Can you work these out from the model? Positions are in its coordinate system, mm. A direction names the side the tool comes from. Round coordinates to 2 decimals unless told otherwise and drop trailing zeros. Loops run counter-clockwise (first coordinate to the right, second up) from the corner with the lowest first, then second, coordinate; pieces in that order, holes last. Notation, with made-up numbers: (-1, -22) -> (33, -22) arc R27 ccw to (33, -2) -> close; hole circle Ø8 at (9, -21). An arc over 180 degrees is marked (long way). Write each question's results on one line, items separated by ' | '.
from build123d import *

# Parameters (mm, degrees)
EXTRUDE_1_DEPTH     = 25
FILLET_1_R          = 8
SKETCH_2_R          = 1.65
CUT_EXTRUDE_1_DEPTH = 137.034003102
SKETCH_3_R          = 1.6
CUT_EXTRUDE_2_DEPTH = 131.794686436


with BuildPart() as part:
    # 草图1 → 凸台-拉伸1 (new, symmetric)
    with BuildSketch(Plane.XY):
        Polygon((0, 0), (0, 119.5), (15, 119.5), (15, 6), (60, 6), (60, 0), align=None)
    extrude(amount=EXTRUDE_1_DEPTH, both=True)

    # 圆角1
    # the kernel refuses this fillet: 8 mm, written as the material it takes off along each edge
    with BuildSketch(Plane(origin=(0, 119.5, 45), x_dir=(0, -1, 0), z_dir=(0, 0, -1)), Plane(origin=(0, 0, -45), x_dir=(0, 1, 0), z_dir=(0, 0, 1))) as fillet_1_piece_1:
        with BuildLine():
            CenterArc((FILLET_1_R, -FILLET_1_R), FILLET_1_R, 90, 90)
            Line((0, -FILLET_1_R), (-FILLET_1_R * 0.02, -FILLET_1_R))
            Line((-FILLET_1_R * 0.02, -FILLET_1_R), (-FILLET_1_R * 0.02, FILLET_1_R * 0.02))
            Line((-FILLET_1_R * 0.02, FILLET_1_R * 0.02), (FILLET_1_R, FILLET_1_R * 0.02))
            Line((FILLET_1_R, FILLET_1_R * 0.02), (FILLET_1_R, 0))
        make_face()
    extrude(amount=90, mode=Mode.SUBTRACT)
    with BuildSketch(Plane(origin=(60, 0, -44.364916731), x_dir=(0, 1, 0), z_dir=(0, 0, 1))) as fillet_1_piece_2:
        with BuildLine():
            CenterArc((8, 7.745966692), FILLET_1_R, 180, 75.522487814)
            Line((0, 7.745966692), (-0.16, 7.745966692))
            Line((-0.16, 7.745966692), (-0.16, 0))
            Line((-0.16, 0), (0, -0.16))
            ThreePointArc((0, -0.16), (3, -0.16), (5.96, -0.154919334))
            Line((5.96, -0.154919334), (6, 0))
        make_face()
    extrude(amount=88.729833462, mode=Mode.SUBTRACT)

    # 草图2 → 切除-拉伸1 (cut, through all)
    with BuildSketch(Plane.ZY):
        with Locations((10, 12)):
            Circle(SKETCH_2_R)
        with Locations((-10, 12)):
            Circle(SKETCH_2_R)
    extrude(amount=-CUT_EXTRUDE_1_DEPTH, mode=Mode.SUBTRACT)

    # 草图3 → 切除-拉伸2 (cut, through all)
    with BuildSketch(Plane(origin=(0, 6, 0), x_dir=(1, 0, 0), z_dir=(0, 1, 0))):
        with Locations(Location((21, -20, 0), (0, 0, 270))):
            Circle(SKETCH_3_R)
        with Locations(Location((21, 0, 0), (0, 0, 270))):
            Circle(SKETCH_3_R)
    extrude(amount=-CUT_EXTRUDE_2_DEPTH, mode=Mode.SUBTRACT)


solid = part.part
1. On a 3-axis mill with a long thin cutter (end or side, diameter ignored), from which of +Z, -Z, +X, -X, +Y, -Y can I reach the whole of each face in a straight line? I mean faces 4 (the face through (37, 6, 0)), 5 (the face through (22.08, 3.04, 18.82)). Say none if no direction works.
Final values:
face 4: +Z, -Z, +X, +Y | face 5: +Y, -Y
2. Will these pins go through, and if not, where does the flat tip stop? pin 1 (2.5 mm diameter, centred on y = 12, z = -10, fed in from +X); pin 2 (4 mm diameter, centred on x = 50, z = -4.5, fed in from +Y); pin 3 (5.5 mm diameter, centred on y = 12, z = 10, fed in from +X).
Final values:
pin 1: through | pin 2: y = 6 | pin 3: x = 15
3. Please list where these lines run through material, in increasing order: line 1 (Y direction, x = 9, z = -10); line 2 (X direction, y = 45.5, z = -12); line 3 (Y direction, x = 21, z = -21.5). Write a range as from..to.
Final values:
line 1: 0..10.35, 13.65..119.5 | line 2: 0..15 | line 3: 0..6
4. If we section it at A-A (z = 10): List the corners of the cut face in (x, y) for me.
Final values:
outline: (0, 8) arc R8 ccw to (8, 0) -> (52.25, 0) arc R8 ccw to (60, 6) -> (15, 6) -> (15, 10.35) -> (0, 10.35) -> close; (0, 13.65) -> (15, 13.65) -> (15, 119.5) -> (8, 119.5) arc R8 ccw to (0, 111.5) -> close
5. If we section it at D-D (y = 40): List the corners of the cut face in (x, z) for me.
Final values:
outline: (0, -25) -> (15, -25) -> (15, 25) -> (0, 25) -> close
6. If we section it at B-B (x = 21): List the corners of the cut face in (y, z) for me, then the cut area to 3 significant figures.
Final values:
outline: (0, -25) -> (6, -25) -> (6, -1.6) -> (0, -1.6) -> close; (0, 1.6) -> (6, 1.6) -> (6, 18.4) -> (0, 18.4) -> close; (0, 21.6) -> (6, 21.6) -> (6, 25) -> (0, 25) -> close | area: 262 mm2
7. We'd pull the mould along Y, two halves only. Please class faces 1 (the face through (57.094, 1.631, -0.35)), 2 (the face through (7.395, 10.536, 10.761)), 3 (the face through (11, 119.5, 0)): pulls with the +Y half, pulls with the -Y half, needs draft (parallel to the pull), parting line crosses it, or undercut.
Final values:
face 1: pulls with the -Y half | face 2: undercut | face 3: pulls with the +Y half
8. If we section it at C-C (z = 4): List the corners of the cut face in (x, y) for me, then the cut area to 3 significant figures.
Final values:
outline: (0, 8) arc R8 ccw to (8, 0) -> (52.25, 0) arc R8 ccw to (60, 6) -> (15, 6) -> (15, 119.5) -> (8, 119.5) arc R8 ccw to (0, 111.5) -> close | area: 2,020 mm2
